Part model, mm, in its own coordinate system. Face numbers are marked on the shaded views. A direction names the side the tool comes from. Coordinates: 2 decimals unless noted, no trailing zeros. Loops run counter-clockwise (first coordinate to the right, second up) from the corner with the lowest first, then second, coordinate; pieces in that order, holes last.
```python
from build123d import *

# Parameters (mm, degrees)
SKETCH1_R           = 10
BOSS_EXTRUDE3_DEPTH = 3
BOSS_EXTRUDE4_DEPTH = 10


with BuildPart() as part:
    # Sketch1 → Boss-Extrude3 (new body)
    with BuildSketch(Plane.XY):
        with Locations((-13.989793671, 22.267450219)):
            Circle(SKETCH1_R)
    extrude(amount=BOSS_EXTRUDE3_DEPTH)

    # Sketch3 → Boss-Extrude4 (add)
    with BuildSketch(Plane(origin=(0, 0, 0), x_dir=(-1, 0, 0), z_dir=(0, 0, -1))):
        with BuildLine():
            ThreePointArc((21.489793671, 22.267450219), (19.29309453, 27.570751078), (13.989793671, 29.767450219))
            Line((13.989793671, 29.767450219), (13.989793671, 14.767450219))
            ThreePointArc((13.989793671, 14.767450219), (19.29309453, 16.96414936), (21.489793671, 22.267450219))
        make_face()
        with BuildLine():
            Line((13.989793671, 14.767450219), (13.989793671, 29.767450219))
            ThreePointArc((13.989793671, 29.767450219), (6.489793671, 22.267450219), (13.989793671, 14.767450219))
        make_face()
    extrude(amount=BOSS_EXTRUDE4_DEPTH)

    # Fillet1: read off the stored shape, not the designer's step
    # Fillet1 outline → Fillet1 (revolve, cut)
    with BuildSketch(Plane(origin=(-13.989793671, 22.267450219, 0), x_dir=(1, 0, 0), z_dir=(0, -1, 0))):
        with BuildLine():
            Line((7.5, -10), (7.5, -7.5))
            ThreePointArc((7.5, -7.5), (6.767766953, -9.267766953), (5, -10))
            Line((5, -10), (7.5, -10))
        make_face()
    revolve(axis=Axis((-13.989793671, 22.267450219, 0), (0, 0, 1)), mode=Mode.SUBTRACT)


solid = part.part
```
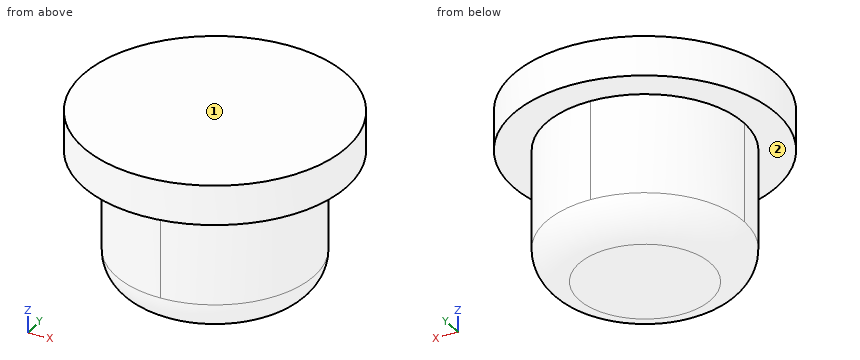
Q1. Tool access for the marked faces 1 and 2: list every direction of +Z, -Z, +X, -X, +Y, -Y with a clear straight run to the whole face (end or side of a thin tool).
Q2. Saw through at A-A (z = -0.75). List the corners of the cut face in (x, y), plus the area to 3 significant figures.
Q3. Probe line 1 (Z direction, x = -7.75, y = 27.5); line 2 (Y direction, x = -14, z = -6.5); line 3 (Y direction, x = -22.25, z = 1.5). List the from-to ranges inside material, lowest first.
Q4. Saw through at B-B (z = 1). List the corners of the cut face in (x, y), plus the area to 3 significant figures.
Q5. Drop flat-ended pins along their axis: P1, Ø8, axis at x = -10, y = 18.5, coming from the -Z side; P2, Ø1, axis at y = 19.5, z = -8, coming from the +X side; P3, Ø1.5, axis at y = 25.5, z = 1.5, coming from the +X side; P4, Ø3, axis at y = 26, z = -7, coming from the +X side. Give the stop position or say it passes through.
Q6. Saw through at C-C (z = -8.25). List the corners of the cut face in (x, y).
Checked values:
1. face 1: +Z, +X, -X, +Y, -Y
1. face 2: -Z
2. outline: circle Ø15 at (-13.99, 22.27)
2. area: 177 mm2
3. line 1: z = 0 to 3
3. line 2: y = 14.77 to 29.77
3. line 3: y = 16.63 to 27.9
4. outline: circle Ø20 at (-13.99, 22.27)
4. area: 314 mm2
5. P1: stops at z = -10
5. P2: stops at x = -6.87
5. P3: stops at x = -4.3
5. P4: stops at x = -6.83
6. outline: circle Ø14.77 at (-13.99, 22.27)
